Verification items for this drawing (mm, ordinates from the low corner). A direction names the side the tool comes from. Round coordinates to 2 decimals unless told otherwise and drop trailing zeros. Loops run counter-clockwise (first coordinate to the right, second up) from the corner with the lowest first, then second, coordinate; pieces in that order, holes last. Notation, with made-up numbers: M 80.5,1.5 L 133.5,1.5 A27 cw 133.5,40.5 Z; hole C 48.5,-37.5 d8. An arc over 180 degrees is marked long. One line per item, written item: value.
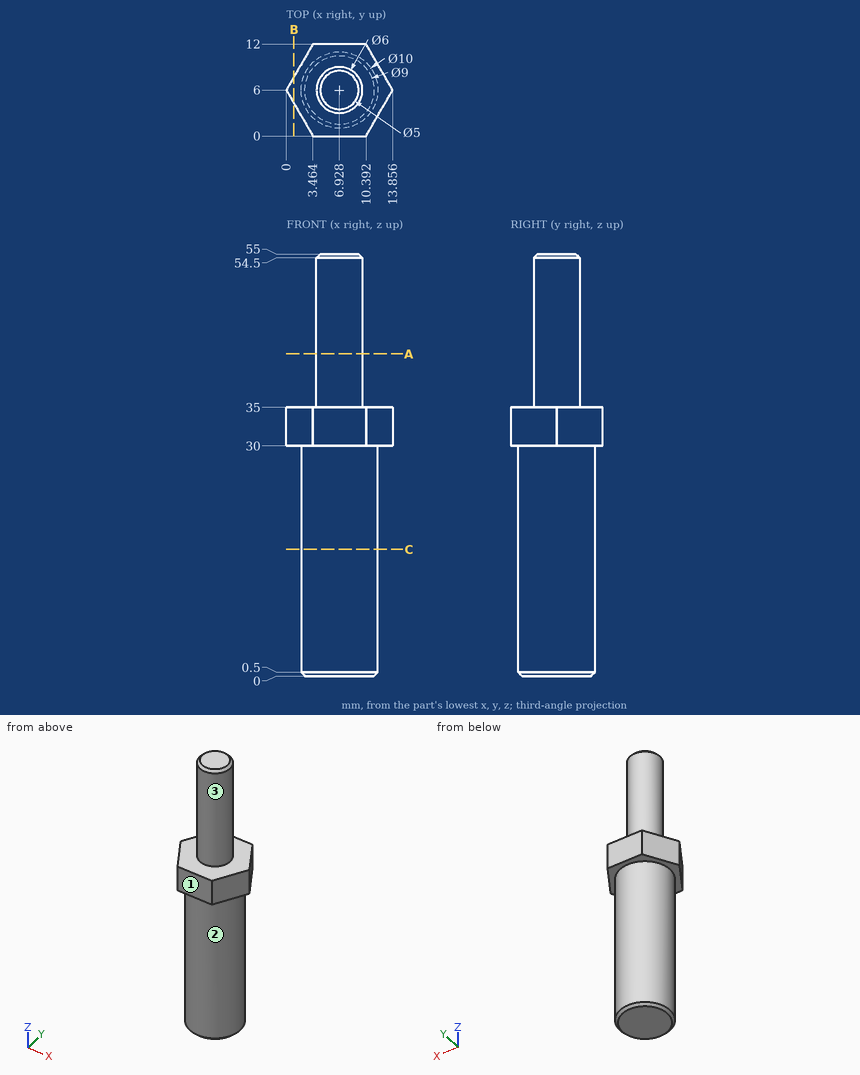
(1) Sectioned sample at C-C on z = 16.5. Enter the section's corners in (x, y).
Completed:
outline: C 6.93,6 d10
(2) Thickness scan on L1, parallel to X at y = 6.25, z = 46; L2, parallel to Z at x = 12, y = 3; L3, parallel to Z at x = 3.25, y = 3.75. Record the ranges inside material, lowest first. Write a range as from..to.
Completed:
L1: x = 3.94..9.92
L2: z = 30..35
L3: z = 0..35
(3) Sectioned sample at A-A on z = 42. Enter the section's corners in (x, y).
Completed:
outline: C 6.93,6 d6
(4) Depth check by flat-ended pin: pin 1 Ø2 at (y, z) = (8.5, 40.5) entering from -X; pin 2 Ø1 at (x, z) = (4.5, 23) entering from +Y; pin 3 Ø2 at (x, z) = (3.5, 40) entering from +Y. Enter the tip coordinate at first touch or a pass-through.
Completed:
pin 1: stops at x = 4.33
pin 2: stops at y = 10.61
pin 3: stops at y = 7.76
(5) Tool access check on the marked faces 1, 2 and 3. Record the directions out of +Z, -Z, +X, -X, +Y, -Y that give a thin tool (end or side, any length) a straight path to the whole face; none if there is none.
Completed:
face 1: +Z, -Z, +X, -X, -Y
face 2: -Z
face 3: +Z
(6) Sectioned sample at B-B on x = 1. Enter the section's corners in (y, z), and give its area (3 significant figures).
Completed:
outline: M 4.27,30 L 7.73,30 L 7.73,35 L 4.27,35 Z
area: 17.3 mm^2
